Autodesk Inventor part; units mm, degrees
ref_plane "Work Plane1" through (-57.15, 3.175, 0) normal (1, 0, 0) x (0, 0, -1)
ref_plane "YZ Plane" through (0, 0, 0) normal (1, 0, 0) x (0, 1, 0)
ref_plane "XZ Plane" through (0, 0, 0) normal (0, 1, 0) x (-1, 0, 0)
sketch "Sketch1" plane through (0, 0, 0) normal (0, 0, 1) x (1, 0, 0)
  line L0 (0, 0) -> (-114.3, 0)
  line L1 (-114.3, 0) -> (-114.3, 63.5)
  line L2 (-114.3, 63.5) -> (0, 63.5)
  line L3 (0, 63.5) -> (0, 0)
  dimension "d7" = 114.3
  dimension "d8" = 63.5
extrude "Extrusion1" add sketch "Sketch1" along normal blind 6.35
sketch "Sketch2" plane through (0, 0, 6.35) normal (0, 0, 1) x (1, 0, 0)
  line L0 (0, 0) -> (0, 63.5)
  line L1 (-114.3, 63.5) -> (-114.3, 0)
  line L2 (-114.3, 0) -> (0, 0)
  line L3 (0, 63.5) -> (-114.3, 63.5)
sketch "Sketch3" plane through (0, 0, 6.35) normal (0, 0, 1) x (1, 0, 0)
  line L0 (-110.6716, 35.2666) -> (-52.0005, 35.2666) construction
  line L1 (-52.0005, 35.2666) -> (-52.0005, 28.3217) construction
  line L2 (-52.0005, 28.3217) -> (-110.6716, 28.3217) construction
  line L3 (-110.6716, 28.3217) -> (-110.6716, 35.2666) construction
  line L4 (-114.3, 63.5) -> (-114.3, 0)
  line L5 (-107.8928, 19.0941) -> (-105.5257, 34.5523)
  line L6 (-105.5257, 34.5523) -> (-89.1412, 34.5523)
  line L7 (-89.1412, 34.5523) -> (-88.8942, 36.0343)
  spline S0 degree 2 poles (-88.8942, 36.0343) (-88.8119, 36.693) (-88.9766, 37.8663) (-89.3882, 38.7514) (-89.9852, 39.2659) (-90.3145, 39.2659) knots 0 0 0 1 2 3 4 4 4
  line L8 (-90.3145, 39.2659) -> (-107.1929, 39.2659)
  spline S1 degree 2 poles (-107.1929, 39.2659) (-106.9048, 40.3157) (-106.2667, 42.8063) (-105.9168, 43.8561) knots 0 0 0 1 2 2 2
  line L9 (-105.9168, 43.8561) -> (-105.6492, 44.4941)
  line L10 (-105.6492, 44.4941) -> (-87.3505, 44.4941)
  spline S2 degree 2 poles (-87.3505, 44.4941) (-86.6301, 44.4941) (-85.0451, 43.7737) (-83.7484, 42.3123) (-82.925, 40.1922) (-82.9662, 38.7308) knots 0 0 0 1 2 3 4 4 4
  line L11 (-82.9662, 38.7308) -> (-85.9714, 19.0941)
  line L12 (-85.9714, 19.0941) -> (-91.4878, 19.0941)
  line L13 (-91.4878, 19.0941) -> (-89.9234, 29.3241)
  line L14 (-89.9234, 29.3241) -> (-100.8121, 29.3241)
  line L15 (-100.8121, 29.3241) -> (-102.3764, 19.0941)
  line L16 (-102.3764, 19.0941) -> (-107.8928, 19.0941)
  spline S3 degree 2 poles (-81.5048, 39.2659) (-81.2166, 40.3157) (-80.5785, 42.8063) (-80.2492, 43.8561) knots 0 0 0 1 2 2 2
  line L17 (-80.2492, 43.8561) -> (-79.961, 44.4941)
  line L18 (-79.961, 44.4941) -> (-56.7017, 44.4941)
  spline S4 degree 2 poles (-56.7017, 44.4941) (-56.9693, 43.4444) (-57.628, 40.9538) (-57.9779, 39.904) knots 0 0 0 1 2 2 2
  line L19 (-57.9779, 39.904) -> (-58.2455, 39.2659)
  line L20 (-58.2455, 39.2659) -> (-66.0054, 39.2659)
  line L21 (-66.0054, 39.2659) -> (-69.0724, 19.0941)
  line L22 (-69.0724, 19.0941) -> (-74.5887, 19.0941)
  line L23 (-74.5887, 19.0941) -> (-71.5218, 39.2659)
  line L24 (-71.5218, 39.2659) -> (-81.5048, 39.2659)
  spline S5 degree 2 poles (-58.3072, 24.8575) (-58.369, 23.3961) (-57.525, 21.276) (-56.2283, 19.8146) (-54.6434, 19.0941) (-53.9435, 19.0941) knots 0 0 0 1 2 3 4 4 4
  line L25 (-53.9435, 19.0941) -> (-37.168, 19.0941)
  line L26 (-37.168, 19.0941) -> (-33.2983, 44.4941)
  line L27 (-33.2983, 44.4941) -> (-38.8147, 44.4941)
  line L28 (-38.8147, 44.4941) -> (-41.8816, 24.3223)
  line L29 (-41.8816, 24.3223) -> (-50.9795, 24.3223)
  spline S6 degree 2 poles (-50.9795, 24.3223) (-51.2882, 24.3223) (-51.8852, 24.8369) (-52.3174, 25.7014) (-52.4821, 26.8541) (-52.3792, 27.5334) knots 0 0 0 1 2 3 4 4 4
  line L30 (-52.3792, 27.5334) -> (-49.7857, 44.4941)
  line L31 (-49.7857, 44.4941) -> (-55.302, 44.4941)
  line L32 (-55.302, 44.4941) -> (-58.3072, 24.8575)
  line L33 (-31.2605, 44.4941) -> (-35.1508, 19.0941)
  line L34 (-35.1508, 19.0941) -> (-29.6344, 19.0941)
  line L35 (-29.6344, 19.0941) -> (-27.0409, 36.0755)
  spline S7 degree 2 poles (-27.0409, 36.0755) (-26.444, 35.0257) (-25.1472, 32.4116) (-23.8093, 29.5094) (-22.4302, 26.463) (-21.7716, 24.9604) knots 0 0 0 1 2 3 4 4 4
  line L36 (-21.7716, 24.9604) -> (-21.6892, 24.9604)
  spline S8 degree 2 poles (-21.6892, 24.9604) (-20.5777, 26.463) (-18.2518, 29.5505) (-16.0493, 32.4528) (-13.9498, 35.0257) (-13.0236, 36.0755) knots 0 0 0 1 2 3 4 4 4
  line L37 (-13.0236, 36.0755) -> (-15.6171, 19.0941)
  line L38 (-15.6171, 19.0941) -> (-10.1007, 19.0941)
  line L39 (-10.1007, 19.0941) -> (-6.231, 44.4941)
  line L40 (-6.231, 44.4941) -> (-12.2002, 44.4941)
  spline S9 degree 2 poles (-12.2002, 44.4941) (-13.6205, 43.2797) (-17.202, 39.1424) (-19.0545, 36.8783) knots 0 0 0 1 2 2 2
  line L41 (-19.0545, 36.8783) -> (-20.1249, 35.6021)
  spline S10 degree 2 poles (-20.1249, 35.6021) (-21.7716, 38.8543) (-24.221, 43.3209) (-25.2913, 44.4941) knots 0 0 0 1 2 2 2
  line L42 (-25.2913, 44.4941) -> (-31.2605, 44.4941)
  point P0 (0, 0)
extrude "Extrusion2" add sketch "Sketch3" along normal blind 1.143
fillet "Fillet2" radius 3.175 4 edges at (-114.3, 63.5, 3.175) (-114.3, 0, 3.175) (0, 0, 3.175) (0, 63.5, 3.175)
sketch "Sketch4" plane through (0, 0, 6.35) normal (0, 0, 1) x (1, 0, 0)
  point P0 (0, 0)
sketch "Sketch5" plane through (0, 0, 6.35) normal (0, 0, 1) x (1, 0, 0)
  point P0 (0, 0)
sketch "Sketch6" plane through (0, 0, 6.35) normal (0, 0, 1) x (1, 0, 0)
  point P0 (0, 0)
ref_plane "Work Plane1" through (-57.15, 3.175, 0) normal (1, 0, 0) x (0, 0, -1)
sketch "Sketch7" plane through (-111.125, 63.5, 0) normal (0, 1, 0) x (1, 0, 0)
  line L0 (107.95, -6.35) -> (0, -6.35)
  line L1 (107.95, 0) -> (0, 0)
  line L2 (0, -6.35) -> (0, -3.175)
  line L3 (0, -6.35) -> (0, 0)
  line L4 (0, 0) -> (0, -6.35)
  line L5 (0, -6.35) -> (0, -3.5306)
  line L6 (0, -3.5306) -> (6.985, -3.5306)
  line L7 (6.985, -3.5306) -> (11.8618, -3.5306)
  line L8 (11.8618, -3.5306) -> (11.8618, -1.651)
  line L9 (11.8618, -1.651) -> (6.985, -1.651)
  line L10 (6.985, -1.651) -> (6.985, -3.5306)
  point P0 (111.125, 0)
  dimension "d24" = 4.8768
  dimension "d25" = 1.8796
  dimension "d26" = 2.8194
  dimension "d27" = 6.985
extrude "Extrusion3" cut sketch "Sketch7" against normal blind 9.652
sketch "Sketch8" plane through (-111.125, 0, 0) normal (0, -1, 0) x (1, 0, 0)
  line L0 (0, 0) -> (0, 6.35)
  line L1 (6.985, 3.5306) -> (6.985, 1.651)
  line L2 (11.8618, 1.651) -> (11.8618, 3.5306)
  line L3 (6.985, 1.651) -> (11.8618, 1.651)
  line L4 (11.8618, 1.651) -> (11.8618, 3.5306)
  line L5 (11.8618, 3.5306) -> (6.985, 3.5306)
  line L6 (6.985, 3.5306) -> (6.985, 1.651)
  line L7 (0, 0) -> (107.95, 0)
  point P0 (111.125, 0)
extrude "Extrusion4" cut sketch "Sketch8" against normal blind 9.652
mirror "Mirror1" about plane through (-57.15, 3.175, 0) normal (1, 0, 0) of "Extrusion3"
mirror "Mirror2" about plane through (-57.15, 3.175, 0) normal (1, 0, 0) of "Extrusion4"
properties part number "custom plate"
Design review of the part built by this model. Coordinates are the model's own, in mm. A direction names the side the tool comes from. Give positions to 0.01 mm unless a question says otherwise; leave off trailing zeros. Write each loop counter-clockwise with the first axis right and the second up, starting at its lowest first coordinate (ties: lowest second). Pieces come first, ordered by that corner, then holes. Notation, with made-up numbers: M -6,-15.75 L 20,-15.75 A21 ccw 20,2.25 Z; hole C -5,72.5 d6. An arc over 180 degrees is marked long. Answer as a JSON object with one key per item and string values. Group by question number.
1) We need section B-B (x = -93). Give the boundary of the cut face in (y, z).
2) Clearance check with flat-ended pins moving along their axes: pin 1 Ø0.9 at (x, z) = (-99, 7) entering from -Y; pin 2 Ø0.9 at (x, z) = (-63.5, 7) entering from -Y; pin 3 Ø2 at (x, y) = (-67, 25.5) entering from +Z. State where each tip first meets the part, or that it passes through.
3) Tool access review of faces 1 (the face through (-73.077, 29.039, 6.913)), 2 (the face through (-40.327, 34.549, 6.913)), 3 (the face through (-28.356, 27.466, 6.913)), 4 (the face through (-106.726, 26.715, 6.913)), 5 (the face through (-56, 0, 3)): name each direction out of +Z, -Z, +X, -X, +Y, -Y from which nothing blocks a thin tool from reaching the whole face with its end or side.
4) For line 1 along Z through (x, y) = (-88, 56.5); line 2 along Y through (x, z) = (-62.5, 6.75), list the stretches that pass through material, from the lowest coordinate up.
5) We need section D-D (x = -78). Give the boundary of the cut face in (y, z).
6) We need section A-A (y = 8). Give the boundary of the cut face in (x, z).
7) We need section C-C (y = 50). Give the boundary of the cut face in (x, z), and give its area (3 significant figures).
8) Mouldability with a two-part tool opening along Z and no side actions: class faces 6 (the face through (-13, 5, 1.651)), 7 (the face through (-40, 29, 7.493)), 8 (the face through (-13, 59, 3.531)), 9 (the face through (-114.3, 31, 3)) as released by +Z, released by -Z, zero draft, split by the parting line, or undercut.
Answer key:
{
 "1": {"outline": "M 0,0 L 63.5,0 L 63.5,6.35 L 44.49,6.35 L 44.49,7.49 L 39.27,7.49 L 39.27,6.35 L 34.55,6.35 L 34.55,7.49 L 29.32,7.49 L 29.32,6.35 L 0,6.35 Z"},
 "2": {"pin 1": "stops at y = 29.32", "pin 2": "stops at y = 39.27", "pin 3": "stops at z = 6.35"},
 "3": {"face 1": "+Z", "face 2": "+Z, +Y", "face 3": "+Z, -Y", "face 4": "+Z, -X", "face 5": "+Z, -Z, +X, -X, -Y"},
 "4": {"line 1": "z = 0 to 6.35", "line 2": "y = 39.27 to 44.49"},
 "5": {"outline": "M 0,0 L 63.5,0 L 63.5,6.35 L 44.49,6.35 L 44.49,7.49 L 39.27,7.49 L 39.27,6.35 L 0,6.35 Z"},
 "6": {"outline": "M -114.3,0 L 0,0 L 0,6.35 L -114.3,6.35 Z; hole M -104.14,1.65 L -99.26,1.65 L -99.26,3.53 L -104.14,3.53 Z; hole M -15.04,1.65 L -10.16,1.65 L -10.16,3.53 L -15.04,3.53 Z"},
 "7": {"outline": "M -114.3,0 L 0,0 L 0,6.35 L -114.3,6.35 Z", "area": "726 mm²"},
 "8": {"face 6": "undercut", "face 7": "released by +Z", "face 8": "undercut", "face 9": "zero draft"}
}
